Geometry check sheet. Reference: the model listing, model coordinates, mm. Round coordinates to 2 decimals unless told otherwise and drop trailing zeros. Use a Markdown table: item, result.
```python
from build123d import *

# Parameters (mm, degrees)
F0_W     = 14
F0_H     = 21
F0_W_2   = 6
F0_H_2   = 1.7
F1_DEPTH = 15
F1_TAPER = 3
F2_DEPTH = 12
F2_TAPER = -3
F3_R     = 2


with BuildPart() as f1:
    # F0 (on Top) → F1 (new body)
    with BuildSketch(Plane.XY):
        Rectangle(F0_W, F0_H)
        Rectangle(F0_W_2, F0_H_2, mode=Mode.SUBTRACT)
        Rectangle(F0_W_2, F0_H_2)
    extrude(amount=F1_DEPTH, taper=F1_TAPER)

    # F0 (on Top) → F2 (cut)
    with BuildSketch(Plane.XY):
        Rectangle(F0_W_2, F0_H_2)
    extrude(amount=F2_DEPTH, taper=F2_TAPER, mode=Mode.SUBTRACT)

    # F3
    f3_edges = [f1.edges().sort_by_distance(p)[0] for p in [
        (-6.606942, 10.106942, 7.5),
        (-6.606942, -10.106942, 7.5),
        (6.606942, 10.106942, 7.5),
        (6.606942, -10.106942, 7.5),
        (6.213883, 0, 15),
        (0, -9.713883, 15),
        (0, 9.713883, 15),
        (-6.213883, 0, 15),
    ]]
    fillet(f3_edges, radius=F3_R)


with BuildPart() as f5:
    # F4 (on Top) → F5 (revolve)
    with BuildSketch(Plane.XY):
        with BuildLine():
            Line((0, 15), (0, -15))
            add(Edge.make_bspline(
                [(0, -15), (8.0832192465, -15), (8.0832192465, 0), (8.0832192465, 15), (0, 15)],
                knots=[3.1415926536, 3.1415926536, 3.1415926536, 4.7123889804, 4.7123889804, 6.2831853072, 6.2831853072, 6.2831853072], degree=2, weights=[1, 0.7071067812, 1, 0.7071067812, 1]))
        make_face()
    revolve(axis=Axis((0, -0.4179980606, 0), (0, -1, 0)))


with BuildPart() as f5_1:
    # F6: moved
    add(f5.part.moved(Location((0, 0, 21.9))))


with BuildPart() as f1_1:
    add(f1.part)

    # F7: cut F5
    add(f5_1.part, mode=Mode.SUBTRACT)


solid = f1_1.part
```
(1) Release check for a two-part mould opening along Y. For faces 1 (the face through (0, 0, 12)), 2 (the face through (-5.708, -0.109, 14.436)), 3 (the face through (-0.07, 10.16, 6.46)), 4 (the face through (6.05, -9.58, 6.66)) record: +Y half, -Y half, draft (parallel to the pull), parting line (faces both ways), or undercut.
A:
| item | result |
|---|---|
| face 1 | undercut |
| face 2 | draft |
| face 3 | +Y half |
| face 4 | -Y half |
(2) Gauge pin test, flat ends, axial feed: pin 1 Ø1 at (y, z) = (0, 2) entering from -X; pin 2 Ø2 at (x, z) = (3, 7) entering from +Y; pin 3 Ø1 at (x, z) = (0, 2.5) entering from +Y. Record the tip position at first contact, or that the pin passes through.
A:
| item | result |
|---|---|
| pin 1 | stops at x = -6.92 |
| pin 2 | stops at y = 10.19 |
| pin 3 | stops at y = 10.4 |
(3) Thickness scan on line 1 (X direction, y = -0.25, z = 6.25); line 2 (X direction, y = -3.5, z = 13); line 3 (Z direction, x = 0, y = -0.25). Record the ranges inside material, lowest first.
A:
| item | result |
|---|---|
| line 1 | x = -6.67 to -3.33, 3.33 to 6.67 |
| line 2 | x = -6.32 to 6.32 |
| line 3 | z = 12 to 13.82 |
